Here's how the part is built. I have some questions about the finished solid (model axes, mm). A direction names the side the tool comes from. Round coordinates to 2 decimals unless told otherwise and drop trailing zeros. Order: outer loops, then holes, each group sorted by start corner. A loop starts at its lowest first (then second) coordinate and runs counter-clockwise, first axis right, second up. Notation, with made-up numbers: (-25.5, -3) -> (-2.5, -3) arc R11 cw to (-2.5, 10) -> close; hole circle Ø7 at (50, 40.25). An arc over 180 degrees is marked (long way). Use a Markdown table: item, result. Add a question column.
from build123d import *

# Parameters (mm, degrees)
BOSS_EXTRUDE1_DEPTH     = 12.7
CUT_EXTRUDE1_DEPTH      = 26.162
CUT_EXTRUDE1_DEPTH_BACK = 25.4
SKETCH3_W               = 21.105033739
SKETCH3_H               = 30.717467856
SKETCH4_R               = 2.54
CUT_EXTRUDE2_DEPTH      = 50.8
SKETCH9_R               = 4.2291
CUT_EXTRUDE3_DEPTH      = 29.21
SKETCH11_R              = 3.81
CUT_EXTRUDE4_DEPTH      = 12.7
SKETCH12_R              = 2.54
CUT_EXTRUDE5_DEPTH      = 12.7


with BuildPart() as part:
    # Sketch1 → Boss-Extrude1 (new body)
    with BuildSketch(Plane.XY):
        Polygon((0, 0), (44.45, 0), (44.45, 6.35), (0, 82.55), align=None)
    extrude(amount=BOSS_EXTRUDE1_DEPTH)

    # Sketch3 → Cut-Extrude1 (cut, two sides: drawn at the far end of the back side and taken through both)
    with BuildSketch(Plane.XY.offset(-CUT_EXTRUDE1_DEPTH_BACK)):
        Polygon((3.81, 37.067467856), (22.120626117, 37.067467856), (10.4058157, 57.15), (3.81, 57.15), align=None)
        with Locations((14.36251687, 19.168733928)):
            Rectangle(SKETCH3_W, SKETCH3_H)
        Polygon((27.455033739, 3.81), (41.5208157, 3.81), (27.455033739, 27.922769076), align=None)
        Polygon((6.6675, 71.12), (0, 71.12), (0, 82.55), align=None)
    extrude(amount=CUT_EXTRUDE1_DEPTH + CUT_EXTRUDE1_DEPTH_BACK, mode=Mode.SUBTRACT)

    # Sketch4 → Cut-Extrude2 (cut)
    with BuildSketch(Plane.XZ):
        with Locations((33.02, 6.35)):
            Circle(SKETCH4_R)
    extrude(amount=-CUT_EXTRUDE2_DEPTH, mode=Mode.SUBTRACT)

    # Sketch9 → Cut-Extrude3 (cut)
    with BuildSketch(Plane(origin=(0, 3.81, 0), x_dir=(1, 0, 0), z_dir=(0, 1, 0))):
        with Locations(Location((33.02, -6.35, 0), (0, 0, 167.415562146))):
            Circle(SKETCH9_R)
    extrude(amount=CUT_EXTRUDE3_DEPTH, mode=Mode.SUBTRACT)

    # Sketch11 → Cut-Extrude4 (cut)
    with BuildSketch(Plane(origin=(3.81, 0, 0), x_dir=(0, 0, -1), z_dir=(1, 0, 0))):
        with Locations(Location((-6.35, 63.5, 0), (0, 0, 90))):
            Circle(SKETCH11_R)
    extrude(amount=CUT_EXTRUDE4_DEPTH, mode=Mode.SUBTRACT)

    # Sketch12 → Cut-Extrude5 (cut)
    with BuildSketch(Plane(origin=(3.81, 0, 0), x_dir=(0, 0, -1), z_dir=(1, 0, 0))):
        with Locations(Location((-6.35, 63.5, 0), (0, 0, 90))):
            Circle(SKETCH12_R)
    extrude(amount=-CUT_EXTRUDE5_DEPTH, mode=Mode.SUBTRACT)


solid = part.part
(1) I want a section at D-D on y = 43.5. List the corners of the cut face in (x, z) for me, and give its area (3 significant figures).
(2) Please list where these lines run through material, in increasing order: probe 1 along Y at (x, z) = (4.5, 2.5); probe 2 along X at (y, z) = (12, 10); probe 3 along Y at (x, z) = (14, 8.75). Write a range as from..to.
(3) I'm going to push flat-ended pins straight in: P1, Ø6.5, axis at x = 33.02, z = 6.35, coming from the -Y side; P2, Ø6.5, axis at y = 26, z = 8, coming from the +X side; P3, Ø6, axis at y = 64.5, z = 4.5, coming from the +X side; P4, Ø4, axis at y = 32, z = 5, coming from the +X side. Where does each tip first touch, or does it pass through?
(4) If we mould it in two halves opening along Y, with no side actions, what happens to faces 4 (the flat face through (13, 37.067, 6)), 5 (the flat face through (3, 71.12, 6)), 6 (the flat face through (22, 0, 6))? For each: pulls with the +Y half, pulls with the -Y half, needs draft (parallel to the pull), parting line crosses it, or undercut.
(5) I want a section at B-B on x = 33. List the corners of the cut face in (y, z) for me.
(6) I want a section at A-A on z = 6.35. State how many separate pieces and enclosed holes the cut face has, and give its area (3 significant figures).
(7) I want a section at C-C on y = 18.5. List the corners of the cut face in (x, z) for me.
(8) On a 3-axis mill with a long thin cutter (end or side, diameter ignored), from which of +Z, -Z, +X, -X, +Y, -Y can I reach the whole of each face in a straight line? I mean faces 1 (the flat face through (3.81, 63, 9)), 2 (the flat face through (14, 3.81, 6)), 3 (the flat face through (16, 36, 0)). Say none if no direction works.
Output:
| question | item | result |
|---|---|---|
| 1 | outline | (0, 0) -> (3.81, 0) -> (3.81, 12.7) -> (0, 12.7) -> close; (18.37, 0) -> (22.78, 0) -> (22.78, 12.7) -> (18.37, 12.7) -> close |
| 1 | area | 104 mm² |
| 2 | probe 1 | 0..3.81, 34.53..37.07, 57.15..71.12 |
| 2 | probe 2 | 0..3.81, 24.92..27.46, 36.74..41.15 |
| 2 | probe 3 | 0..3.81, 34.53..37.07, 50.99..58.55 |
| 3 | P1 | y = 0 |
| 3 | P2 | x = 34.27 |
| 3 | P3 | x = 11.99 |
| 3 | P4 | x = 30.1 |
| 4 | face 4 | undercut |
| 4 | face 5 | pulls with the +Y half |
| 4 | face 6 | pulls with the -Y half |
| 5 | outline | (0, 0) -> (3.81, 0) -> (3.81, 3.81) -> (0, 3.81) -> close; (0, 8.89) -> (3.81, 8.89) -> (3.81, 12.7) -> (0, 12.7) -> close; (18.42, 0) -> (25.98, 0) -> (25.98, 2.12) -> (18.42, 2.12) -> close; (18.42, 10.58) -> (25.98, 10.58) -> (25.98, 12.7) -> (18.42, 12.7) -> close |
| 6 | separate pieces | 3 |
| 6 | enclosed holes | 2 |
| 6 | area | 711 mm² |
| 7 | outline | (0, 0) -> (3.81, 0) -> (3.81, 12.7) -> (0, 12.7) -> close; (24.92, 0) -> (27.46, 0) -> (27.46, 12.7) -> (24.92, 12.7) -> close; (32.95, 0) -> (37.36, 0) -> (37.36, 12.7) -> (32.95, 12.7) -> (32.95, 10.58) arc R4.23 cw (long way) to (32.95, 2.12) -> close |
| 8 | face 1 | +X |
| 8 | face 2 | +Z, -Z |
| 8 | face 3 | -Z, +X, -X, +Y, -Y |
